from build123d import *

# Parameters (mm, degrees)
SKETCH_1_W           = 30
SKETCH_1_H           = 17
EXTRUDE_1_DEPTH      = 10
SKETCH_2_W           = 14
SKETCH_2_H           = 7
CUT_EXTRUDE_1_DEPTH  = 12
FILLET_1_R           = 3
SKETCH_4_R           = 2
EXTRUDE_2_DEPTH      = 5
EXTRUDE_3_DEPTH      = 1
EXTRUDE_3_DEPTH_BACK = 18


with BuildPart() as part:
    # 草图1 → 凸台-拉伸1 (new body)
    with BuildSketch(Plane(origin=(0, 0, 0), x_dir=(1, 0, 0), z_dir=(0, 1, 0))):
        with Locations((15, 8.5)):
            Rectangle(SKETCH_1_W, SKETCH_1_H)
    extrude(amount=EXTRUDE_1_DEPTH)

    # 草图2 → 切除-拉伸1 (cut)
    with BuildSketch(Plane.ZY):
        with Locations((-8.5, 5)):
            Rectangle(SKETCH_2_W, SKETCH_2_H)
    extrude(amount=-CUT_EXTRUDE_1_DEPTH, mode=Mode.SUBTRACT)

    # 圆角1
    fillet_1_edges = [part.edges().sort_by_distance(p)[0] for p in [
        (30, 10, -8.5),
        (30, 0, -8.5),
        (30, 5, -17),
        (30, 5, 0),
    ]]
    fillet(fillet_1_edges, radius=FILLET_1_R)

    # 草图4 → 凸台-拉伸2 (add)
    with BuildSketch(Plane(origin=(30, 0, 0), x_dir=(0, 0, -1), z_dir=(1, 0, 0))):
        with Locations(Location((8.5, 5, 0), (0, 0, 270))):
            Circle(SKETCH_4_R)
    extrude(amount=EXTRUDE_2_DEPTH)

    # 草图5 → 凸台-拉伸3 (add, two sides: drawn at the far end of the back side and taken through both)
    with BuildSketch(Plane.XY.offset(-EXTRUDE_3_DEPTH_BACK)):
        Polygon((36.704530888, 9.683160127), (33.295469112, 0.316839873), (89.677026359, -20.204368726), (93.086088136, -10.838048473), align=None)
    extrude(amount=EXTRUDE_3_DEPTH + EXTRUDE_3_DEPTH_BACK)


solid = part.part
The listing builds one solid part. Answer for the finished solid, in the listing's coordinates (mm). A direction names the side the tool comes from. Give positions to 0.01 mm unless a question says otherwise; leave off trailing zeros. Write each loop counter-clockwise with the first axis right and the second up, starting at its lowest first coordinate (ties: lowest second). Pieces come first, ordered by that corner, then holes.
1) For a pull along Y with two mould halves and no side action, classify faces 4 (the face through (6, 5, -15.5)), 5 (the face through (63, -6, -18)), 6 (the face through (65.29, -0.72, -8.63)), 7 (the face through (13, 0, -9)) as pulls with the +Y half, pulls with the -Y half, needs draft (parallel to the pull), parting line crosses it, or undercut.
2) Section A-A (z = -4.5) is taken. Write down the section's boundary in (x, y).
3) Find the intervals of material crossed by L1, parallel to Y at x = 21, z = -13.25; L2, parallel to Y at x = 43.5, z = -0.5; L3, parallel to Z at x = 32, y = 4, in increasing order.
4) Section C-C (x = 45.5) is taken. Write down the section's boundary in (y, z), and give its area (3 significant figures).
5) Section B-B (y = -18) is taken. Write down the section's boundary in (x, z), and give its area (3 significant figures).
6) Given P1, Ø5.5, axis at x = 3, y = 5.5, coming from the +Z side; P2, Ø2, axis at x = 49.5, z = -2.5, coming from the -Y side; P3, Ø9.5, axis at x = 4, z = -8, coming from the -Y side; P4, Ø8, axis at x = 49, y = -10.5, coming from the +Z side, each flat-ended and moving along its own axis, determine where each tip first touches the part or whether it passes through.
7) A tool of negligible diameter and unlimited length cuts with its end or side. For faces 1 (the face through (32.465, 6.998, -8.588)), 2 (the face through (13, 5, -17)), 3 (the face through (12, 5, -9)), from which of +Z, -Z, +X, -X, +Y, -Y can it reach the whole face along a straight path? Write none if from no direction.
Response:
1. face 4: undercut
1. face 5: needs draft
1. face 6: pulls with the +Y half
1. face 7: pulls with the -Y half
2. outline: (0, 0) - (27, 0) arc R3 ccw to (30, 3) - (30, 7) arc R3 ccw to (27, 10) - (0, 10) - (0, 8.5) - (12, 8.5) - (12, 1.5) - (0, 1.5) - close; (33.3, 0.32) - (89.68, -20.2) - (93.09, -10.84) - (36.7, 9.68) - close
3. L1: y = 0 to 10
3. L2: y = -3.4 to 7.21
3. L3: z = -10.23 to -6.77
4. outline: (-4.13, -18) - (6.48, -18) - (6.48, 1) - (-4.13, 1) - close
4. area: 202 mm2
5. outline: (83.62, -18) - (90.48, -18) - (90.48, 1) - (83.62, 1) - close
5. area: 130 mm2
6. P1: stops at z = 0
6. P2: stops at y = -5.95
6. P3: stops at y = 0
6. P4: passes through
7. face 1: none
7. face 2: -Z, -X, +Y, -Y
7. face 3: -X
